Input: part model. Units: mm. Frame: model coordinates. A direction names the side the tool comes from. Give positions to 0.01 mm unless a question says otherwise; leave off trailing zeros. Order: outer loops, then holes, each group sorted by start corner. A loop starts at its lowest first (then second) coordinate and runs counter-clockwise, first axis right, second up. Notation, with made-up numbers: M -18,-26 L 39,-26 A20 cw 39,-20 Z; hole C 3,-24 d5. An arc over 180 degrees is marked long. Use a Markdown table: item, result.
from build123d import *

# Parameters (mm, degrees)
BOSS_EXTRUDE1_START = 4
BOSS_EXTRUDE1_DEPTH = 5
ANTENNAHOLSTER1_R   = 2.43625
BOSS_EXTRUDE2_DEPTH = 40
ANTENNAHOLSTER2_R   = 2.43625
BOSS_EXTRUDE3_DEPTH = 40


with BuildPart() as part:
    # Trapezoid1 → Boss-Extrude1 (new body)
    with BuildSketch(Plane(origin=(0, 0, 0), x_dir=(1, 0, 0), z_dir=(0, 1, 0)).offset(BOSS_EXTRUDE1_START)):
        Polygon((-114.335639632, -37.176097112), (-96.835639632, -19.676097112), (-61.835639632, -19.676097112), (-44.335639632, -37.176097112), align=None)
    extrude(amount=BOSS_EXTRUDE1_DEPTH)

    # AntennaHolster1 → Boss-Extrude2 (add)
    with BuildSketch(Plane(origin=(-40.755868372, 0, 40.755868372), x_dir=(-0.7071067811865513, 0, -0.7071067811865438), z_dir=(0.7071067811865438, 0, -0.7071067811865513))):
        with BuildLine():
            Line((5.062561066, 11.55), (5.062561066, 4))
            Line((5.062561066, 4), (29.811298407, 4))
            Line((29.811298407, 4), (29.811298407, 11.55))
            Line((29.811298407, 11.55), (22.423126617, 11.55))
            ThreePointArc((22.423126617, 11.55), (15.707633336, 21.13), (8.992140056, 11.55))
            Line((8.992140056, 11.55), (5.062561066, 11.55))
        make_face()
        with Locations((15.707633336, 13.98625)):
            Circle(ANTENNAHOLSTER1_R, mode=Mode.SUBTRACT)
    extrude(amount=BOSS_EXTRUDE2_DEPTH)

    # AntennaHolster2 → Boss-Extrude3 (add)
    with BuildSketch(Plane(origin=(-38.57977126, 0, -38.57977126), x_dir=(-0.7071067811865462, 0, 0.7071067811865489), z_dir=(-0.7071067811865489, 0, -0.7071067811865462))):
        with BuildLine():
            Line((82.38623914, 11.55), (82.38623914, 4))
            Line((82.38623914, 4), (107.134976481, 4))
            Line((107.134976481, 4), (107.134976481, 11.55))
            Line((107.134976481, 11.55), (103.736913224, 11.55))
            ThreePointArc((103.736913224, 11.55), (97.021419943, 21.13), (90.305926663, 11.55))
            Line((90.305926663, 11.55), (82.38623914, 11.55))
        make_face()
        with Locations((97.021419943, 13.98625)):
            Circle(ANTENNAHOLSTER2_R, mode=Mode.SUBTRACT)
    extrude(amount=BOSS_EXTRUDE3_DEPTH)


solid = part.part
1) Cut plane D-D on x = -70.5. Return loops of the section in (y, z), and give its area (3 significant figures).
Response values:
| item | result |
|---|---|
| outline | M 4,19.68 L 9,19.68 L 9,37.18 L 4,37.18 Z |
| area | 87.5 mm² |
2) Mould query, pull axis X, two halves, no side actions, for faces 4 (the face through (-80, 6, 19.676)), 5 (the face through (-32, 11.55, 22)), 6 (the face through (-24.679, 10.782, 0.264)). Classes: released by +X, released by -X, zero draft, split by the parting line, or undercut.
Response values:
| item | result |
|---|---|
| face 4 | undercut |
| face 5 | zero draft |
| face 6 | released by +X |
3) Cut plane C-C on z = 14.5. State how many separate pieces and enclosed holes the cut face has, and give its area (3 significant figures).
Response values:
| item | result |
|---|---|
| separate pieces | 2 |
| enclosed holes | 2 |
| area | 799 mm² |
4) First-contact query: pin 1 Ø4 at (x, y) = (-55, 8) entering from -Z; pin 2 Ø5 at (y, z) = (17, 19) entering from -X; pin 3 Ø19.5 at (x, z) = (-80, 29.5) entering from +Y; pin 4 Ø10 at (x, z) = (-90.5, 11) entering from +Y. Flat tips, straight axial feed; report the tip coordinate or a pass-through.
Response values:
| item | result |
|---|---|
| pin 1 | stops at z = 10.84 |
| pin 2 | stops at x = -130.19 |
| pin 3 | stops at y = 9 |
| pin 4 | passes through |
5) Reachability of faces 1 (the face through (-38.054, 21.127, 15.569)), 2 (the face through (-47.89, 7.72, 5.73)), 3 (the face through (-52.96, 16.5, 28.55)) from +Z, -Z, +X, -X, +Y, -Y: full face, straight path, thin tool, end or side. Return the list, or none.
Response values:
| item | result |
|---|---|
| face 1 | none |
| face 2 | -Z, +Y, -Y |
| face 3 | +Z, +Y |
6) Material intervals for line 1 (X direction, y = 16, z = 17); line 2 (X direction, y = 15.5, z = 26); line 3 (Y direction, x = -34.5, z = -3.5), sorted ascending. Write a range as from..to.
Response values:
| item | result |
|---|---|
| line 1 | x = -129.9..-122.15, -118.27..-110.52, -48.91..-41.15, -37.27..-29.52 |
| line 2 | x = -121.08..-113.91, -108.51..-103.16, -55.51..-50.91, -45.51..-38.34 |
| line 3 | y = 4..11.55 |
7) Cut plane A-A on y = 18. Return loops of the section in (x, z).
Response values:
| item | result |
|---|---|
| outline | M -139.65,5.92 L -131.29,-2.44 L -103.01,25.85 L -111.36,34.2 Z; M -56.04,25.47 L -27.76,-2.81 L -19.4,5.54 L -47.68,33.83 Z |
8) Cut plane B-B on y = 6.25. Return loops of the section in (x, z).
Response values:
| item | result |
|---|---|
| outline | M -142.62,8.89 L -125.12,-8.61 L -96.84,19.68 L -61.84,19.68 L -33.55,-8.61 L -16.05,8.89 L -44.34,37.18 L -114.34,37.18 Z |
